from build123d import *

# Parameters (mm, degrees)
BOSS_EXTRUDE1_DEPTH               = 2.5
TAP_DRILL_FOR_M2_TAP2_D           = 1.6
TAP_DRILL_FOR_M2_TAP2_CSINK_D     = 1.65
TAP_DRILL_FOR_M2_TAP2_CSINK_ANGLE = 90


# Read off the part's stored shape, not the designer's step: Tap Drill for M2 Tap1
with BuildPart() as part:
    # Sketch1 → Boss-Extrude1 (new, symmetric)
    with BuildSketch(Plane(origin=(0, 0, 0), x_dir=(1, 0, 0), z_dir=(0, 1, 0))):
        Polygon((55, 45), (45, 45), (45, 40), (35, 40), (35, 45), (25, 45), (25, 40), (15, 40), (15, 45), (5, 45), (5, 40), (-5, 40), (-5, 45), (-15, 45), (-15, 40), (-25, 40), (-25, 45), (-35, 45), (-35, 40), (-45, 40), (-45, 45), (-55, 45), (-55, 40), (-55, 35), (-60, 35), (-60, 25), (-55, 25), (-55, 15), (-60, 15), (-60, 5), (-55, 5), (-55, -5), (-60, -5), (-60, -15), (-55, -15), (-55, -25), (-60, -25), (-60, -35), (-55, -35), (-55, -40), (-55, -45), (-45, -45), (-45, -40), (-35, -40), (-35, -45), (-25, -45), (-25, -40), (-15, -40), (-15, -45), (-5, -45), (-5, -40), (5, -40), (5, -45), (15, -45), (15, -40), (25, -40), (25, -45), (35, -45), (35, -40), (45, -40), (45, -45), (55, -45), (55, -40), (55, -35), (60, -35), (60, -25), (55, -25), (55, -15), (60, -15), (60, -5), (55, -5), (55, 5), (60, 5), (60, 15), (55, 15), (55, 25), (60, 25), (60, 35), (55, 35), (55, 40), align=None)
    extrude(amount=BOSS_EXTRUDE1_DEPTH, both=True)

    # Tap Drill for M2 Tap1 outline → Tap Drill for M2 Tap1 (revolve, cut)
    with BuildSketch(Plane(origin=(3, 0, -27.5), x_dir=(1, 0, 0), z_dir=(0, 0, 1))):
        Polygon((0.8, -2.475), (0.8, 2.5), (0, 2.5), (0, -2.5), (0.825, -2.5), align=None)
    revolve(axis=Axis((3, 0, -27.5), (0, 1, 0)), mode=Mode.SUBTRACT)

    # Tap Drill for M2 Tap1 2 outline → Tap Drill for M2 Tap1 2 (revolve, cut)
    with BuildSketch(Plane(origin=(-3, 0, -27.5), x_dir=(1, 0, 0), z_dir=(0, 0, 1))):
        Polygon((0.8, -2.475), (0.8, 2.5), (0, 2.5), (0, -2.5), (0.825, -2.5), align=None)
    revolve(axis=Axis((-3, 0, -27.5), (0, 1, 0)), mode=Mode.SUBTRACT)

    # Tap Drill for M2 Tap2 (through all)
    with Locations(Plane(origin=(0, -2.5, 0), x_dir=(-1, 0, 0), z_dir=(0, -1, 0))):
        with Locations((-7.5, 15.5), (7.5, 15.5), (-7.5, -16.5), (7.5, -16.5)):
            CounterSinkHole(TAP_DRILL_FOR_M2_TAP2_D / 2, TAP_DRILL_FOR_M2_TAP2_CSINK_D / 2, counter_sink_angle=TAP_DRILL_FOR_M2_TAP2_CSINK_ANGLE)


solid = part.part
Geometry check sheet. Reference: the model listing, model coordinates, mm. A direction names the side the tool comes from. Give positions to 0.01 mm unless a question says otherwise; leave off trailing zeros. Write each loop counter-clockwise with the first axis right and the second up, starting at its lowest first coordinate (ties: lowest second). Pieces come first, ordered by that corner, then holes. Notation, with made-up numbers: M 62,78 L 73,78 A16 cw 73,96 Z; hole C 11,-20 d9. An arc over 180 degrees is marked long. One line per question, with ' | ' between items.
1. Set-up check for faces 1 (the face through (45, 0, -43)), 2 (the face through (60, 0, 30)), 3 (the face through (25, 0, 42)), 4 (the face through (-58, 0, 15)), 5 (the face through (58, 0, -15)): record each of +Z, -Z, +X, -X, +Y, -Y from which the full face is reachable in a straight line by a thin tool's end or side.
Ans:
face 1: -Z, +Y, -Y | face 2: +Z, -Z, +X, +Y, -Y | face 3: +Z, +Y, -Y | face 4: -X, +Y, -Y | face 5: +X, +Y, -Y
2. Cross-section at A-A (y = 0.95). Count the separate pieces of the cut face and the enclosed holes in it, plus the area to 3 significant figures.
Ans:
separate pieces: 1 | enclosed holes: 6 | area: 9,790 mm2
3. Gauge pin test, flat ends, axial feed: pin 1 (1.5 mm diameter, centred on y = -1, z = 41.5, fed in from -X); pin 2 (1.5 mm diameter, centred on y = -1.5, z = 17.5, fed in from +X); pin 3 (1 mm diameter, centred on x = -23, y = 0.5, fed in from +Z). Record the tip position at first contact, or that the pin passes through.
Ans:
pin 1: x = -55 | pin 2: x = 55 | pin 3: z = 40
4. Scan lines: line 1 along X through (y, z) = (0.7, -27.5); line 2 along Z through (x, y) = (-7.5, 0.95); line 3 along Z through (x, y) = (36.5, -0.6). Record each from-to range of solid material in increasing order. Write a range as from..to.
Ans:
line 1: -60..-3.8, -2.2..2.2, 3.8..60 | line 2: -45..-16.3, -14.7..15.7, 17.3..45 | line 3: -40..40
5. Cross-section at B-B (x = -41). Enter the section's corners in (y, z), plus the area to 3 significant figures.
Ans:
outline: M -2.5,-40 L 2.5,-40 L 2.5,40 L -2.5,40 Z | area: 400 mm2
6. Mould release check, pull along X, two halves, no side actions. Record for faces 6 (the face through (55, 0, 40)), 7 (the face through (35, 0, -42)), 8 (the face through (57, 0, -5)): released by +X, released by -X, zero draft, split by the parting line, or undercut.
Ans:
face 6: released by +X | face 7: undercut | face 8: zero draft
